Check sheet for the modelled part. Datum: model origin and axes. Units: mm. Round coordinates to 2 decimals unless told otherwise and drop trailing zeros. Loops run counter-clockwise (first coordinate to the right, second up) from the corner with the lowest first, then second, coordinate; pieces in that order, holes last. Notation, with made-up numbers: M -16.5,-13 L 18.5,-13 A18 ccw 18.5,17 Z; hole C 42.5,-18.75 d11. An arc over 180 degrees is marked long. Write item = value, one per line. Start each with the question number.
(1) Cross-section at B-B on x = -114.5. Record the boundary of the cut face in (y, z).
(2) Cross-section at C-C on z = 99. Record the boundary of the cut face in (x, y), plus the area to 3 significant figures.
(3) Cross-section at A-A on z = 63.5. Record the boundary of the cut face in (x, y), plus the area to 3 significant figures.
(4) Go/stop test with a flat-tipped pin: P1, Ø4, axis at x = 8, y = -82, coming from the -Z side. Record where the tip stops, or that it passes through.
(5) Scan lines: L1, parallel to Y at x = -17, z = 51; L2, parallel to X at y = -158, z = 74. Record each from-to range of solid material in increasing order. Write a range as from..to.
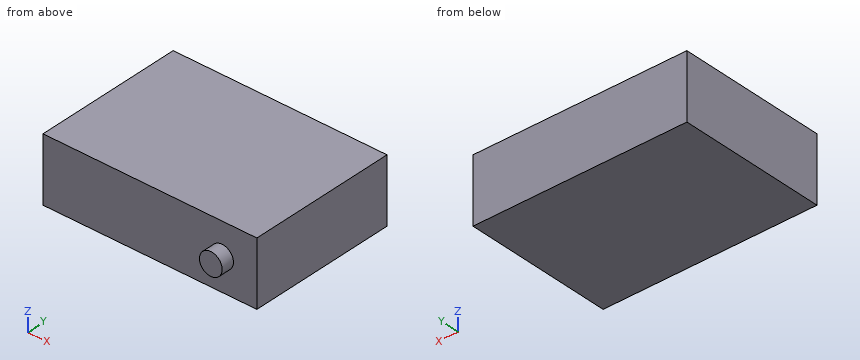
from build123d import *

# Parameters (mm, degrees)
F0_W     = 419.1
F0_H     = 292.1
F1_DEPTH = 127
F2_R     = 22.225
F3_DEPTH = 25.4


with BuildPart() as f1:
    # F0 (on Top) → F1 (new body)
    with BuildSketch(Plane.XY):
        Rectangle(F0_W, F0_H)
    extrude(amount=F1_DEPTH)

    # F2 (on face) → F3 (join)
    with BuildSketch(Plane.XZ.offset(146.05)):
        with Locations((141.425312, 63.5)):
            Circle(F2_R)
    extrude(amount=F3_DEPTH)


solid = f1.part
Result:
q1.outline = M -146.05,0 L 146.05,0 L 146.05,127 L -146.05,127 Z
q2.outline = M -209.55,-146.05 L 209.55,-146.05 L 209.55,146.05 L -209.55,146.05 Z
q2.area = 122,000 mm^2
q3.outline = M -209.55,-146.05 L 119.2,-146.05 L 119.2,-171.45 L 163.65,-171.45 L 163.65,-146.05 L 209.55,-146.05 L 209.55,146.05 L -209.55,146.05 Z
q3.area = 124,000 mm^2
q4.P1 = 0
q5.L1 = -146.05..146.05
q5.L2 = 121.84..161.01
